Can you work these out from the model? Positions are in its coordinate system, mm. A direction names the side the tool comes from. Coordinates: 2 decimals unless noted, no trailing zeros. Order: outer loops, then holes, each group sorted by start corner. A loop starts at its lowest first (then second) coordinate and runs counter-clockwise, first axis right, second up. Notation, with made-up numbers: (35.25, 7.5) -> (49.25, 7.5) arc R28 ccw to (49.25, 31.5) -> close; hole circle Ø8 at (40.5, 0.25). An arc over 180 degrees is marked (long way). Answer as CSV lines item,"result".
from build123d import *

# Parameters (mm, degrees)
SKETCH3_R           = 2.7813
BOSS_EXTRUDE3_DEPTH = 2.54
SKETCH4_W           = 3.81
SKETCH4_H           = 40.386
BOSS_EXTRUDE4_DEPTH = 20.32
SKETCH5_W           = 40.386
SKETCH5_H           = 1.524
BOSS_EXTRUDE5_DEPTH = 5.08
SKETCH6_W           = 40.386
SKETCH6_H           = 1.524
BOSS_EXTRUDE6_DEPTH = 5.08
SKETCH7_W           = 40.64
SKETCH7_H           = 20.32
CUT_EXTRUDE1_DEPTH  = 5.08
SKETCH11_W          = 40.64
SKETCH11_H          = 35.306
BOSS_EXTRUDE7_DEPTH = 2.9718
BOSS_EXTRUDE8_DEPTH = 35.306
SKETCH8_W           = 14.986
SKETCH8_H           = 20.32
CUT_EXTRUDE2_DEPTH  = 41.64
CUT_EXTRUDE3_DEPTH  = 36.306
SKETCH14_R          = 3.81
SKETCH14_R_2        = 2.7813
BOSS_EXTRUDE9_DEPTH = 2.54
CUT_EXTRUDE4_DEPTH  = 23.86


with BuildPart() as part:
    # Sketch3 → Boss-Extrude3 (new body)
    with BuildSketch(Plane(origin=(0, 0, 0), x_dir=(1, 0, 0), z_dir=(0, 1, 0))):
        Polygon((-11.517251908, 12.440983784), (29.122748092, 12.440983784), (29.122748092, -34.564151764), (29.122748092, -42.169016216), (18.885256114, -42.169016216), (-11.517251908, -42.169016216), align=None)
        with Locations((3.240148092, -37.089016216)):
            Circle(SKETCH3_R, mode=Mode.SUBTRACT)
        with Locations((14.365348092, -37.089016216)):
            Circle(SKETCH3_R, mode=Mode.SUBTRACT)
    extrude(amount=BOSS_EXTRUDE3_DEPTH)

    # Sketch4 → Boss-Extrude4 (add)
    with BuildSketch(Plane.XZ):
        with Locations((-9.612251908, 7.752016216)):
            Rectangle(SKETCH4_W, SKETCH4_H)
        with Locations((27.217748092, 7.752016216)):
            Rectangle(SKETCH4_W, SKETCH4_H)
    extrude(amount=BOSS_EXTRUDE4_DEPTH)

    # Sketch5 → Boss-Extrude5 (add)
    with BuildSketch(Plane(origin=(-7.707251908, 0, 0), x_dir=(0, 0, -1), z_dir=(1, 0, 0))):
        with Locations((-7.752016216, -19.558)):
            Rectangle(SKETCH5_W, SKETCH5_H)
    extrude(amount=BOSS_EXTRUDE5_DEPTH)

    # Sketch6 → Boss-Extrude6 (add)
    with BuildSketch(Plane.ZY.offset(-25.312748092)):
        with Locations((7.752016216, -19.558)):
            Rectangle(SKETCH6_W, SKETCH6_H)
    extrude(amount=BOSS_EXTRUDE6_DEPTH)

    # Sketch7 → Cut-Extrude1 (cut)
    with BuildSketch(Plane.XY.offset(27.945016216)):
        with Locations((8.802748092, -10.16)):
            Rectangle(SKETCH7_W, SKETCH7_H)
    extrude(amount=-CUT_EXTRUDE1_DEPTH, mode=Mode.SUBTRACT)

    # Sketch11 → Boss-Extrude7 (add)
    with BuildSketch(Plane.XZ):
        with Locations((8.802748092, 5.212016216)):
            Rectangle(SKETCH11_W, SKETCH11_H)
    extrude(amount=BOSS_EXTRUDE7_DEPTH)

    # Sketch12 → Boss-Extrude8 (add)
    with BuildSketch(Plane.XY.offset(22.865016216)):
        Polygon((-7.707251908, -18.796), (-2.593407451, -16.66881978), (-2.627251908, -18.796), align=None)
        Polygon((20.232748092, -18.796), (20.232748092, -16.66881978), (25.312748092, -18.796), align=None)
    extrude(amount=-BOSS_EXTRUDE8_DEPTH)

    # Sketch8 → Cut-Extrude2 (cut, through all)
    with BuildSketch(Plane(origin=(29.122748092, 0, 0), x_dir=(0, 0, -1), z_dir=(1, 0, 0))):
        with Locations((-5.212016216, -10.16)):
            Rectangle(SKETCH8_W, SKETCH8_H)
    extrude(amount=-CUT_EXTRUDE2_DEPTH, mode=Mode.SUBTRACT)

    # Sketch13 → Cut-Extrude3 (cut, through all)
    with BuildSketch(Plane.XY.offset(22.865016216)):
        Polygon((-2.618031664, -18.216492377), (-7.660745747, -20.32), (-2.627251908, -20.32), (-2.627251908, -18.796), align=None)
        Polygon((20.232748092, -18.294602636), (20.232748092, -20.32), (25.312748092, -20.32), align=None)
    extrude(amount=-CUT_EXTRUDE3_DEPTH, mode=Mode.SUBTRACT)

    # Sketch14 → Boss-Extrude9 (add)
    with BuildSketch(Plane.XZ):
        with Locations((3.240148092, 37.089016216)):
            Circle(SKETCH14_R)
        with Locations((3.240148092, 37.089016216)):
            Circle(SKETCH14_R_2, mode=Mode.SUBTRACT)
        with Locations((14.365348092, 37.089016216)):
            Circle(SKETCH14_R)
        with Locations((14.365348092, 37.089016216)):
            Circle(SKETCH14_R_2, mode=Mode.SUBTRACT)
    extrude(amount=-BOSS_EXTRUDE9_DEPTH)

    # Sketch15 → Cut-Extrude4 (cut, through all)
    with BuildSketch(Plane(origin=(0, 2.54, 0), x_dir=(1, 0, 0), z_dir=(0, 1, 0))):
        Polygon((18.885256114, -39.476616216), (13.678256114, -42.169016216), (29.122748092, -42.169016216), (29.122748092, -34.183083779), align=None)
    extrude(amount=-CUT_EXTRUDE4_DEPTH, mode=Mode.SUBTRACT)


solid = part.part
Q1. If I drill on line 1 (Z direction, x = -8, y = -5); line 2 (X direction, y = -4.25, z = 20); line 3 (Y direction, x = -5, z = 38), over which ranges is the centre line in solid material (lowest first)?
Solution:
line 1,"-12.44 to -2.28, 12.71 to 22.87"
line 2,"-11.52 to -7.71, 25.31 to 29.12"
line 3,"0 to 2.54"
Q2. We'd pull the mould along X, two halves only. Please class faces 1 (the flat face through (9, -1, -12.441)), 2 (the flat face through (29.123, 1, 6)), 3 (the flat face through (25.313, -11, 18)): pulls with the +X half, pulls with the -X half, needs draft (parallel to the pull), parting line crosses it, or undercut.
Solution:
face 1,"needs draft"
face 2,"pulls with the +X half"
face 3,"undercut"
Q3. Imagine slicing it at D-D (z = -6). List the corners of the cut face in (x, y) for me.
Solution:
outline,"(-11.52, -20.32) -> (-7.66, -20.32) -> (-2.62, -18.22) -> (-2.59, -16.67) -> (-7.71, -18.8) -> (-7.71, -2.97) -> (25.31, -2.97) -> (25.31, -18.8) -> (20.23, -16.67) -> (20.23, -18.29) -> (25.31, -20.32) -> (29.12, -20.32) -> (29.12, 2.54) -> (-11.52, 2.54) -> close"
Q4. For P1, Ø12, axis at x = 11, z = 8, coming from the -Y side; P2, Ø12, axis at y = -17.5, z = -1.5, coming from the +X side; P3, Ø1, axis at x = 16, z = 0, coming from the -Y side; P4, Ø2, axis at x = 14.5, y = -3.5, coming from the +Z side (3 decimals), each with a flat end and sliding along its axis, tell me the tip position at first contact or that it passes through.
Solution:
P1,"y = -2.97"
P2,"x = 29.12"
P3,"y = 0"
P4,"z = 22.865"
Q5. Which directions (+Z, -Z, +X, -X, +Y, -Y) give clear straight access to the entire face, cutting with the end or side of a thin tool? Please do faces 4 (the flat face through (9, 0, 5)), 5 (the flat face through (-7.707, -11, 18)), 6 (the flat face through (20.233, -17, 18)), 7 (the flat face through (10, -2, 22.865)).
Solution:
face 4,"+X, -X, -Y"
face 5,"+Z, -Z"
face 6,"+Z, -Z, -Y"
face 7,"+Z, +X, -X, -Y"
Q6. Imagine slicing it at B-B (x = -1.5). List the corners of the cut face in (y, z) for me.
Solution:
outline,"(-2.97, -12.44) -> (2.54, -12.44) -> (2.54, 42.17) -> (0, 42.17) -> (0, 22.87) -> (-2.97, 22.87) -> (-2.97, 12.71) -> (0, 12.71) -> (0, -2.28) -> (-2.97, -2.28) -> close"
Q7. Imagine slicing it at A-A (y = -14.5). List the corners of the cut face in (x, z) for me.
Solution:
outline,"(-11.52, -12.44) -> (-7.71, -12.44) -> (-7.71, -2.28) -> (-11.52, -2.28) -> close; (-11.52, 12.71) -> (-7.71, 12.71) -> (-7.71, 22.87) -> (-11.52, 22.87) -> close; (25.31, -12.44) -> (29.12, -12.44) -> (29.12, -2.28) -> (25.31, -2.28) -> close; (25.31, 12.71) -> (29.12, 12.71) -> (29.12, 22.87) -> (25.31, 22.87) -> close"
Q8. Imagine slicing it at C-C (x = 16.5). List the corners of the cut face in (y, z) for me, and give its area (3 significant figures).
Solution:
outline,"(-2.97, -12.44) -> (2.54, -12.44) -> (2.54, 35.31) -> (0, 35.31) -> (0, 22.87) -> (-2.97, 22.87) -> (-2.97, 12.71) -> (0, 12.71) -> (0, -2.28) -> (-2.97, -2.28) -> close; (0, 38.87) -> (2.54, 38.87) -> (2.54, 40.71) -> (0, 40.71) -> close"
area,"186 mm2"
